Could you check a few things on this drawing? It's one solid part, dimensions in mm from its lowest x, y, z. A direction names the side the tool comes from. Give positions to 0.01 mm unless a question says otherwise; leave off trailing zeros. Loops run counter-clockwise (first coordinate to the right, second up) from the corner with the lowest first, then second, coordinate; pieces in that order, holes last. Notation, with made-up numbers: (-15.5, -26) -> (-11.5, -26) arc R23 cw to (-11.5, 11) -> close; hole circle Ø6 at (64, 74.5). An arc over 180 degrees is marked (long way). Use CSV: the item, a comma, the result in double quotes.
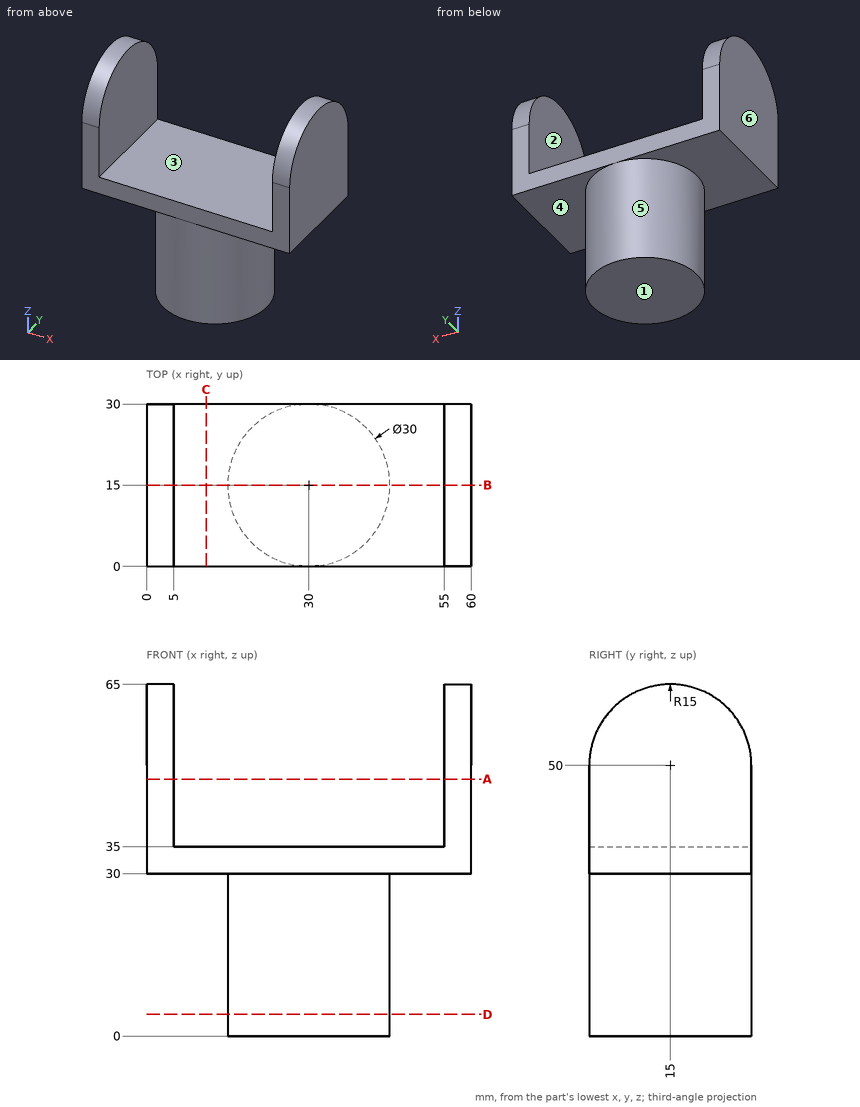
(1) If we section it at B-B, the plane y = 15: Write out the boundary of the cut face in (x, z), then the cut area to 3 significant figures.
Answer sheet:
outline,"(0, 30) -> (15, 30) -> (15, 0) -> (45, 0) -> (45, 30) -> (60, 30) -> (60, 65) -> (55, 65) -> (55, 35) -> (5, 35) -> (5, 65) -> (0, 65) -> close"
area,"1,500 mm2"
(2) If we section it at A-A, the plane z = 47.5: Write out the boundary of the cut face in (x, y), then the cut area to 3 significant figures.
Answer sheet:
outline,"(0, 0) -> (5, 0) -> (5, 30) -> (0, 30) -> close; (55, 0) -> (60, 0) -> (60, 30) -> (55, 30) -> close"
area,"300 mm2"
(3) If we section it at D-D, the plane z = 4: Write out the boundary of the cut face in (x, y), then the cut area to 3 significant figures.
Answer sheet:
outline,"circle Ø30 at (30, 15)"
area,"707 mm2"
(4) We'd pull the mould along X, two halves only. Please class the marked faces 3, 4, 5 and 6: released by +X, released by -X, zero draft, split by the parting line, or undercut.
Answer sheet:
face 3,"undercut"
face 4,"zero draft"
face 5,"split by the parting line"
face 6,"released by -X"
(5) If we section it at C-C, the plane x = 11: Write out the boundary of the cut face in (y, z).
Answer sheet:
outline,"(0, 30) -> (30, 30) -> (30, 35) -> (0, 35) -> close"
(6) Which directions (+Z, -Z, +X, -X, +Y, -Y) give clear straight access to the entire face, cutting with the end or side of a thin tool? Please do the marked faces 1 and 2.
Answer sheet:
face 1,"-Z, +X, -X, +Y, -Y"
face 2,"+Z, +Y, -Y"
(7) If I drill on L1, parallel to X at y = 21.5, z = 37; L2, parallel to Z at x = 15, y = 3.25; L3, parallel to Z at x = 42.5, y = 9.5, over which ranges is the centre line in solid material (lowest first)? Write a range as from..to.
Answer sheet:
L1,"x = 0..5, 55..60"
L2,"z = 30..35"
L3,"z = 0..35"
(8) Will these pins go through, and if not, where does the flat tip stop? pin 1 Ø8 at (x, y) = (42.5, 26.5) entering from -Z; pin 2 Ø3 at (y, z) = (24.5, 10) entering from +X; pin 3 Ø10 at (x, y) = (25, 11) entering from +Z; pin 4 Ø3 at (x, z) = (21, 8.5) entering from -Y.
Answer sheet:
pin 1,"stops at z = 0"
pin 2,"stops at x = 42.69"
pin 3,"stops at z = 35"
pin 4,"stops at y = 2.01"
